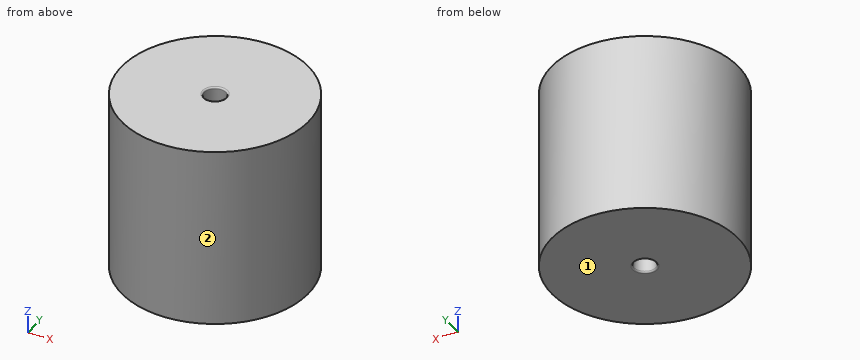
from build123d import *

# Parameters (mm, degrees)
SKETCH21_R           = 30
BOSS_EXTRUDE14_DEPTH = 29
SKETCH24_R           = 3.5
CUT_EXTRUDE1_DEPTH   = 5
SKETCH25_R           = 3.5
CUT_EXTRUDE2_DEPTH   = 5
FILLET1_R            = 0.5


with BuildPart() as part:
    # Sketch21 → Boss-Extrude14 (new body, symmetric)
    with BuildSketch(Plane.XY):
        Circle(SKETCH21_R)
    extrude(amount=BOSS_EXTRUDE14_DEPTH, both=True)

    # Sketch24 → Cut-Extrude1 (cut)
    with BuildSketch(Plane(origin=(0, 0, -29), x_dir=(-1, 0, 0), z_dir=(0, 0, -1))):
        Circle(SKETCH24_R)
    extrude(amount=-CUT_EXTRUDE1_DEPTH, mode=Mode.SUBTRACT)

    # Sketch25 → Cut-Extrude2 (cut)
    with BuildSketch(Plane.XY.offset(29)):
        with Locations(Location((0, 0, 0), (0, 0, 180))):  # turned: the seam where the file's is
            Circle(SKETCH25_R)
    extrude(amount=-CUT_EXTRUDE2_DEPTH, mode=Mode.SUBTRACT)

    # Fillet1
    fillet1_edges = [part.edges().sort_by_distance(p)[0] for p in [
        (3.5, 0, 29),
        (3.5, 0, -29),
    ]]
    fillet(fillet1_edges, radius=FILLET1_R)


solid = part.part
The listing builds one solid part. Answer for the finished solid, in the listing's coordinates (mm). Face numbers are marked on the shaded views. Coordinates: 2 decimals unless noted, no trailing zeros. Order: outer loops, then holes, each group sorted by start corner. A loop starts at its lowest first (then second) coordinate and runs counter-clockwise, first axis right, second up.
Q1. Given P1, Ø4, axis at y = -12, z = 16.5, coming from the -X side; P2, Ø6.5, axis at x = 0, y = 0, coming from the +Z side; P3, Ø5, axis at x = 18, z = -4.5, coming from the -Y side, each flat-ended and moving along its own axis, determine where each tip first touches the part or whether it passes through.
Q2. A cutting plane is placed at A-A, the plane x = 0. Write down the section's boundary in (y, z), and give its area (3 significant figures).
Q3. A cutting plane is placed at C-C, the plane z = 25.5. Write down the section's boundary in (x, y), and give its area (3 significant figures).
Q4. A cutting plane is placed at D-D, the plane z = 9. Write down the section's boundary in (x, y).
Q5. Consider line 1 (Y direction, x = 0, z = 27); line 2 (Y direction, x = 18, z = -18); line 3 (Y direction, x = -6, z = -21). Determine where each line is inside the solid, lowest interval first.
Q6. For a pull along Y with two mould halves and no side action, classify the marked faces 1 and 2 as pulls with the +Y half, pulls with the -Y half, needs draft (parallel to the pull), parting line crosses it, or undercut.
Answers follow:
1. P1: stops at x = -28.28
1. P2: stops at z = 24
1. P3: stops at y = -25.69
2. outline: (-30, -29) - (-4, -29) arc R0.5 ccw to (-3.5, -28.5) - (-3.5, -24) - (3.5, -24) - (3.5, -28.5) arc R0.5 ccw to (4, -29) - (30, -29) - (30, 29) - (4, 29) arc R0.5 ccw to (3.5, 28.5) - (3.5, 24) - (-3.5, 24) - (-3.5, 28.5) arc R0.5 ccw to (-4, 29) - (-30, 29) - close
2. area: 3,410 mm2
3. outline: circle Ø60 at (0, 0); hole circle Ø7 at (0, 0)
3. area: 2,790 mm2
4. outline: circle Ø60 at (0, 0)
5. line 1: y = -30 to -3.5, 3.5 to 30
5. line 2: y = -24 to 24
5. line 3: y = -29.39 to 29.39
6. face 1: needs draft
6. face 2: parting line crosses it
